Part model, mm, in its own coordinate system. A direction names the side the tool comes from. Round coordinates to 2 decimals unless told otherwise and drop trailing zeros. Order: outer loops, then holes, each group sorted by start corner. A loop starts at its lowest first (then second) coordinate and runs counter-clockwise, first axis right, second up. Notation, with made-up numbers: M 70,23 L 129,23 A23 ccw 129,48 Z; hole C 32,60 d8. An arc over 180 degrees is marked long. One line per question, with ' | ' between items.
from build123d import *

# Parameters (mm, degrees)
BASPROSKE_W              = 16
BASPROSKE_H              = 32
TOOTHCUT_DEPTH           = 49
TEETHCUTS_COUNT          = 30
TEETHCUTS_ANGLE          = 348
BORSKE_R                 = 12
BORE_DEPTH               = 50.0000508
SCHIZZO1_R               = 24
SCHIZZO1_R_2             = 17
TAGLIO_ESTRUSIONE1_DEPTH = 3
TAGLIO_ESTRUSIONE2_DEPTH = 48.921417629


with BuildPart() as part:
    # BasProSke → Base-Revolve (revolve)
    with BuildSketch(Plane(origin=(0, 0, 0), x_dir=(1, 0, 0), z_dir=(0, 1, 0)), mode=Mode.PRIVATE) as base_revolve_sk:
        with Locations((8, 16)):
            Rectangle(BASPROSKE_W, BASPROSKE_H)
    revolve(base_revolve_sk.sketch.rotate(Axis((-10, 0, 0), (1, 0, 0)), 180), axis=Axis((-10, 0, 0), (1, 0, 0)))

    # TooCutSke → ToothCut (cut, through all)
    with BuildSketch(Plane(origin=(0, 0, 0), x_dir=(0, 0, -1), z_dir=(1, 0, 0))):
        with BuildLine():
            ThreePointArc((0.918551563, 27.483654488), (0, 27.499), (-0.918551563, 27.483654488))
            ThreePointArc((-0.918551563, 27.483654488), (-1.617208176, 29.787801627), (-2.761784709, 31.906093311))
            ThreePointArc((-2.761784709, 31.906093311), (0, 32.0254), (2.761784709, 31.906093311))
            ThreePointArc((2.761784709, 31.906093311), (1.617208176, 29.787801627), (0.918551563, 27.483654488))
        make_face()
    toothcut = extrude(amount=TOOTHCUT_DEPTH, mode=Mode.SUBTRACT)

    # TeethCuts: ToothCut ×30 about axis
    teethcuts_axis = Axis((-10, 0, 0), (1, 0, 0))
    for i in range(1, TEETHCUTS_COUNT):
        add(toothcut.rotate(teethcuts_axis, i * TEETHCUTS_ANGLE / (TEETHCUTS_COUNT - 1)), mode=Mode.SUBTRACT)

    # BorSke → Bore (cut, symmetric)
    with BuildSketch(Plane(origin=(0, 0, 0), x_dir=(0, 0, -1), z_dir=(1, 0, 0))):
        with Locations(Location((0, 0, 0), (0, 0, 180))):
            Circle(BORSKE_R)
    extrude(amount=BORE_DEPTH, both=True, mode=Mode.SUBTRACT)

    # Schizzo1 → Taglio-Estrusione1 (cut)
    with BuildSketch(Plane(origin=(16, 0, 0), x_dir=(0, 0, -1), z_dir=(1, 0, 0))):
        Circle(SCHIZZO1_R)
        Circle(SCHIZZO1_R_2, mode=Mode.SUBTRACT)
    taglio_estrusione1 = extrude(amount=-TAGLIO_ESTRUSIONE1_DEPTH, mode=Mode.SUBTRACT)

    # Specchia1: Taglio-Estrusione1 across plane
    add(taglio_estrusione1.mirror(Plane(origin=(8, 0, 0), x_dir=(0, 0, 1), z_dir=(1, 0, 0))), mode=Mode.SUBTRACT)

    # Schizzo2 → Taglio-Estrusione2 (cut, through all)
    with BuildSketch(Plane(origin=(16, 0, 0), x_dir=(0, 0, -1), z_dir=(1, 0, 0))):
        with BuildLine():
            Line((4, 15.3), (-4, 15.3))
            Line((-4, 15.3), (-4, 11.313708499))
            ThreePointArc((-4, 11.313708499), (0, 12), (4, 11.313708499))
            Line((4, 11.313708499), (4, 15.3))
        make_face()
    extrude(amount=-TAGLIO_ESTRUSIONE2_DEPTH, mode=Mode.SUBTRACT)


solid = part.part
1) Saw through at B-B (y = 8.5). List the corners of the cut face in (x, z).
The answers:
outline: M 0,-26.15 L 16,-26.15 L 16,-22.44 L 13,-22.44 L 13,-14.72 L 16,-14.72 L 16,-8.47 L 0,-8.47 L 0,-14.72 L 3,-14.72 L 3,-22.44 L 0,-22.44 Z; M 0,8.47 L 16,8.47 L 16,14.72 L 13,14.72 L 13,22.44 L 16,22.44 L 16,26.15 L 0,26.15 L 0,22.44 L 3,22.44 L 3,14.72 L 0,14.72 Z
2) Saw through at A-A (z = 0). List the corners of the cut face in (x, y).
The answers:
outline: M 0,-27.5 L 16,-27.5 L 16,-24 L 13,-24 L 13,-17 L 16,-17 L 16,-12 L 0,-12 L 0,-17 L 3,-17 L 3,-24 L 0,-24 Z; M 0,15.3 L 16,15.3 L 16,17 L 13,17 L 13,24 L 16,24 L 16,27.5 L 0,27.5 L 0,24 L 3,24 L 3,17 L 0,17 Z
3) Saw through at D-D (y = -16). List the corners of the cut face in (x, z).
The answers:
outline: M 0,-24.76 L 16,-24.76 L 16,-17.89 L 13,-17.89 L 13,-5.74 L 16,-5.74 L 16,5.74 L 13,5.74 L 13,17.89 L 16,17.89 L 16,24.76 L 0,24.76 L 0,17.89 L 3,17.89 L 3,5.74 L 0,5.74 L 0,-5.74 L 3,-5.74 L 3,-17.89 L 0,-17.89 Z
4) Probe line 1 (Y direction, x = 1.1, z = 0); line 2 (Z direction, x = 7, y = 0); line 3 (Y direction, x = 10.75, z = 0). List the from-to ranges inside material, lowest first. Write a range as [from, to].
The answers:
line 1: y = [-27.5, -24], [-17, -12], [15.3, 17], [24, 27.5] | line 2: z = [-32, -12], [12, 32] | line 3: y = [-27.5, -12], [15.3, 27.5]
5) Drop flat-ended pins along their axis: pin 1 (5 mm diameter, centred on x = 12, z = -17.5, fed in from -Y); pin 2 (4 mm diameter, centred on x = 5, z = 13.5, fed in from +Y); pin 3 (3 mm diameter, centred on x = 8.5, y = 13.5, fed in from -Z). Give the stop position or say it passes through.
The answers:
pin 1: stops at y = -28.01 | pin 2: stops at y = 28.01 | pin 3: stops at z = -29.47
6) Saw through at C-C (x = 2). Give the number of separate pieces and of enclosed holes in the cut face, plus the area to 3 significant figures.
The answers:
separate pieces: 2 | enclosed holes: 2 | area: 1,380 mm²
7) Which spindle directions (+Z, -Z, +X, -X, +Y, -Y) get a long thin tool onto all of the face, cutting with end or side? Do faces 1 (the face through (7.888, 29.805, -1.625)), 2 (the face through (7.888, -29.743, -1.599)), 3 (the face through (7.89, -25, 16.19)), 4 (the face through (7.888, 4.699, -29.413)). Say none if no direction does.
The answers:
face 1: +X, -X, +Y | face 2: +X, -X, -Y | face 3: +X, -X | face 4: -Z, +X, -X
8) Two-plate mould, pull along Z, no slides. Class faces 5 (the face through (7.89, -10.71, 27.79)), 6 (the face through (7.89, 27.89, 10.64)), 7 (the face through (7.888, -10.755, -27.845)): released by +Z, released by -Z, zero draft, split by the parting line, or undercut.
The answers:
face 5: released by +Z | face 6: undercut | face 7: released by -Z
